Read the model definition and answer for the solid it produces. Units are mm, in the model's axes. A direction names the side the tool comes from. Coordinates: 2 decimals unless noted, no trailing zeros. Write each loop counter-clockwise with the first axis right and the second up, starting at its lowest first coordinate (ties: lowest second). Pieces come first, ordered by that corner, then holes. Notation, with made-up numbers: (-30.75, -3) -> (13.25, -3) arc R21 ccw to (13.25, 21) -> close; hole circle Ø11 at (-12.75, 55). An arc over 180 degrees is marked (long way). Answer as a JSON object with one key per item and string values. Group by question number.
(1) Which of the six approach directions +Z, -Z, +X, -X, +Y, -Y give full straight-line access (tool end or side, diameter ignored) to faces 1 (the face through (14.8, -8, 7.6)), 2 (the face through (22.5, -2, 42)), 3 (the face through (-19.791, 9.986, 10.607)), 4 (the face through (-5, 4, 14)), 5 (the face through (15, 16, 11))?
(2) Find section C-C (z = 10.5). Give the vertices of the cut face in (x, y).
(3) Straight lines are drawn through the part: L1, parallel to Z at x = 15, y = 0.25; L2, parallel to Z at x = 15, y = -5.5; L3, parallel to Z at x = -15, y = 10.2. For each, find the intervals that lie inside material, in ascending order.
(4) For a pull along X with two mould halves and no side action, classify faces 6 (the face through (8, -3, 15)), 7 (the face through (15, -11, 30)), 8 (the face through (-25, 12, 16)) as +X half, -X half, draft (parallel to the pull), parting line (faces both ways), or undercut.
(5) Find section D-D (x = 24.5). Give the vertices of the cut face in (y, z), then the cut area to 3 significant figures.
(6) Flat-ended cylindrical pins translate along their axes: P1, Ø6, axis at x = -19, z = 13.5, coming from the -Y side; P2, Ø4, axis at y = 14, z = 4.5, coming from the -X side; P3, Ø1.5, axis at y = -6, z = 17, coming from the -X side. Find the tip coordinate at first contact, or state that the pin passes through.
(7) Find section B-B (x = 15). Give the vertices of the cut face in (y, z).
from build123d import *

# Parameters (mm, degrees)
CYLINDER007_R         = 3.15
CYLINDER007_DEPTH     = 20
CYLINDER006_R         = 3.15
CYLINDER006_DEPTH     = 20
BOX010_W              = 20
BOX010_H              = 6.3
BOX010_DEPTH          = 1
BOX006_W              = 15
BOX006_H              = 27
BOX006_DEPTH          = 30
CHAMFER002001002_SIZE = 7
FILLET_R              = 12
CHAMFER002001003_SIZE = 4
CYLINDER009_R         = 6.5
CYLINDER009_DEPTH     = 19
CYLINDER008_R         = 3.25
CYLINDER008_DEPTH     = 19
CYLINDER004_R         = 3.15
CYLINDER004_DEPTH     = 36
CYLINDER005_R         = 7
CYLINDER005_DEPTH     = 36
BOX008_W              = 7.8
BOX008_H              = 1
BOX008_DEPTH          = 27
BOX009_W              = 24.5
BOX009_H              = 2
BOX009_DEPTH          = 7.3
CHAMFER002001008_SIZE = 1
BOX011_W              = 33
BOX011_H              = 3.5
BOX011_DEPTH          = 8
BOX012_W              = 20
BOX012_H              = 6
BOX012_DEPTH          = 27
CHAMFER002001007_SIZE = 3
BOX007_W              = 35
BOX007_H              = 23
BOX007_DEPTH          = 27
CHAMFER002001005_SIZE = 3
CHAMFER002001006_SIZE = 8
CHAMFER002001009_SIZE = 3.49
CHAMFER002001010_SIZE = 0.4


with BuildPart() as cylinder007:
    # Cylinder007 → Cylinder007 (new body)
    with BuildSketch(Plane(origin=(0, 0, 1), x_dir=(0, 0, 1), z_dir=(-1, 0, 0))):
        Circle(CYLINDER007_R)
    extrude(amount=CYLINDER007_DEPTH)


with BuildPart() as cylinder006:
    # Cylinder006 → Cylinder006 (new body)
    with BuildSketch(Plane.ZY):
        Circle(CYLINDER006_R)
    extrude(amount=CYLINDER006_DEPTH)


with BuildPart() as fusion003004:
    # Box010 → Box010 (new body)
    with BuildSketch(Plane(origin=(-20, -3.15, 0), x_dir=(1, 0, 0), z_dir=(0, 0, 1))):
        with Locations((10, 3.15)):
            Rectangle(BOX010_W, BOX010_H)
    extrude(amount=BOX010_DEPTH)

    # Fusion003004: union Cylinder007, Cylinder006
    add(cylinder007.part)
    add(cylinder006.part)


with BuildPart() as fusion003004_1:
    # Fusion003004 placement: moved
    add(fusion003004.part.moved(Location((25, 0, 45))))


with BuildPart() as cut004:
    # Box006 → Box006 (new body)
    with BuildSketch(Plane(origin=(7.5, -15, 27), x_dir=(1, 0, 0), z_dir=(0, 0, 1))):
        with Locations((7.5, 13.5)):
            Rectangle(BOX006_W, BOX006_H)
    extrude(amount=BOX006_DEPTH)

    # Chamfer002001002
    chamfer002001002_edges = [cut004.edges().sort_by_distance(p)[0] for p in [
        (15, -15, 27),
    ]]
    chamfer(chamfer002001002_edges, length=CHAMFER002001002_SIZE)

    # Fillet
    fillet_edges = [cut004.edges().sort_by_distance(p)[0] for p in [
        (15, 12, 57),
    ]]
    fillet(fillet_edges, radius=FILLET_R)

    # Chamfer002001003
    chamfer002001003_edges = [cut004.edges().sort_by_distance(p)[0] for p in [
        (15, -15, 57),
    ]]
    chamfer(chamfer002001003_edges, length=CHAMFER002001003_SIZE)

    # Cut004: cut Fusion003004
    add(fusion003004_1.part, mode=Mode.SUBTRACT)


with BuildPart() as cylinder009:
    # Cylinder009 → Cylinder009 (new body)
    with BuildSketch(Plane(origin=(-15, -8, 15), x_dir=(1, 0, 0), z_dir=(0, 1, 0))):
        Circle(CYLINDER009_R)
    extrude(amount=CYLINDER009_DEPTH)


with BuildPart() as cylinder008:
    # Cylinder008 → Cylinder008 (new body)
    with BuildSketch(Plane(origin=(-15, 0, 15), x_dir=(1, 0, 0), z_dir=(0, 1, 0))):
        Circle(CYLINDER008_R)
    extrude(amount=CYLINDER008_DEPTH)


with BuildPart() as cylinder004:
    # Cylinder004 → Cylinder004 (new body)
    with BuildSketch(Plane(origin=(15, -15, 15), x_dir=(1, 0, 0), z_dir=(0, 1, 0))):
        Circle(CYLINDER004_R)
    extrude(amount=CYLINDER004_DEPTH)


with BuildPart() as fusion003008:
    # Cylinder005 → Cylinder005 (new body)
    with BuildSketch(Plane(origin=(15, -34, 15), x_dir=(1, 0, 0), z_dir=(0, 1, 0))):
        Circle(CYLINDER005_R)
    extrude(amount=CYLINDER005_DEPTH)

    # Fusion003008: union Cylinder004
    add(cylinder004.part)


with BuildPart() as cube008:
    # Box008 → Box008 (new body)
    with BuildSketch(Plane(origin=(11.1, 15, 0), x_dir=(1, 0, 0), z_dir=(0, 0, 1))):
        with Locations((3.9, 0.5)):
            Rectangle(BOX008_W, BOX008_H)
    extrude(amount=BOX008_DEPTH)


with BuildPart() as fusion003010:
    # Box009 → Box009 (new body)
    with BuildSketch(Plane(origin=(-25, 14, 11.6), x_dir=(1, 0, 0), z_dir=(0, 0, 1))):
        with Locations((12.25, 1)):
            Rectangle(BOX009_W, BOX009_H)
    extrude(amount=BOX009_DEPTH)

    # Chamfer002001008
    chamfer002001008_edges = [fusion003010.edges().sort_by_distance(p)[0] for p in [
        (-12.75, 16, 11.6),
    ]]
    chamfer(chamfer002001008_edges, length=CHAMFER002001008_SIZE)

    # Fusion003010: union Cube008
    add(cube008.part)


with BuildPart() as cube011:
    # Box011 → Box011 (new body)
    with BuildSketch(Plane(origin=(-25, 11.5, 0), x_dir=(1, 0, 0), z_dir=(0, 0, 1))):
        with Locations((16.5, 1.75)):
            Rectangle(BOX011_W, BOX011_H)
    extrude(amount=BOX011_DEPTH)


with BuildPart() as chamfer002001007:
    # Box012 → Box012 (new body)
    with BuildSketch(Plane(origin=(-25, 9, 0), x_dir=(1, 0, 0), z_dir=(0, 0, 1))):
        with Locations((10, 3)):
            Rectangle(BOX012_W, BOX012_H)
    extrude(amount=BOX012_DEPTH)

    # Chamfer002001007
    chamfer002001007_edges = [chamfer002001007.edges().sort_by_distance(p)[0] for p in [
        (-25, 12, 27),
        (-25, 12, 0),
    ]]
    chamfer(chamfer002001007_edges, length=CHAMFER002001007_SIZE)


with BuildPart() as chamfer002001010:
    # Box007 → Box007 (new body)
    with BuildSketch(Plane(origin=(-5, -8, 0), x_dir=(1, 0, 0), z_dir=(0, 0, 1))):
        with Locations((17.5, 11.5)):
            Rectangle(BOX007_W, BOX007_H)
    extrude(amount=BOX007_DEPTH)

    # Chamfer002001005
    chamfer002001005_edges = [chamfer002001010.edges().sort_by_distance(p)[0] for p in [
        (30, -8, 13.5),
    ]]
    chamfer(chamfer002001005_edges, length=CHAMFER002001005_SIZE)

    # Chamfer002001006
    chamfer002001006_edges = [chamfer002001010.edges().sort_by_distance(p)[0] for p in [
        (-5, -8, 13.5),
    ]]
    chamfer(chamfer002001006_edges, length=CHAMFER002001006_SIZE)

    # Fusion003009: union Chamfer002001007
    add(chamfer002001007.part)

    # Cut005: cut Cube011
    add(cube011.part, mode=Mode.SUBTRACT)

    # Chamfer002001009
    chamfer002001009_edges = [chamfer002001010.edges().sort_by_distance(p)[0] for p in [
        (1.5, 15, 8),
    ]]
    chamfer(chamfer002001009_edges, length=CHAMFER002001009_SIZE)

    # Fusion003011: union Fusion003010
    add(fusion003010.part)

    # Cut006: cut Fusion003008
    add(fusion003008.part, mode=Mode.SUBTRACT)

    # Cut007: cut Cylinder008
    add(cylinder008.part, mode=Mode.SUBTRACT)

    # Cut008: cut Cylinder009
    add(cylinder009.part, mode=Mode.SUBTRACT)

    # Fusion003012: union Cut004
    add(cut004.part)

    # Chamfer002001010
    chamfer002001010_edges = [chamfer002001010.edges().sort_by_distance(p)[0] for p in [
        (8, 13.25, 0),
        (-7, 11.5, 0),
        (-13.5, 9, 0),
        (24.45, 15, 0),
        (30, 5, 0),
        (28.5, -6.5, 0),
        (15, -8, 0),
        (-1, -4, 0),
        (-5, 4.5, 0),
        (18.9, 15.5, 0),
        (11.1, 15.5, 0),
        (15, 16, 0),
        (9.55, 15, 0),
    ]]
    chamfer(chamfer002001010_edges, length=CHAMFER002001010_SIZE)


solid = chamfer002001010.part
Results below:
{
 "1": {"face 1": "-Z, +X, -X, -Y", "face 2": "+Z, +X, +Y, -Y", "face 3": "-Y", "face 4": "+Z, -Z, -X, -Y", "face 5": "+Z, -Z, +X, -X, +Y"},
 "2": {"outline": "(-25, 9) -> (-19.69, 9) -> (-19.69, 11) -> (-10.31, 11) -> (-10.31, 9) -> (-5, 9) -> (-5, 0) -> (3, -8) -> (9.64, -8) -> (9.64, 2) -> (20.36, 2) -> (20.36, -8) -> (27, -8) -> (30, -5) -> (30, 15) -> (18.9, 15) -> (18.9, 16) -> (11.1, 16) -> (11.1, 15) -> (8, 15) -> (8, 14.01) -> (-25, 14.01) -> close"},
 "3": {"L1": "z = 0 to 8, 22 to 41.86, 49.14 to 57", "L2": "z = 0 to 8, 22 to 57", "L3": "z = 0 to 8.5, 21.5 to 27"},
 "4": {"face 6": "undercut", "face 7": "draft", "face 8": "-X half"},
 "5": {"outline": "(-8, 0.4) -> (-7.6, 0) -> (14.6, 0) -> (15, 0.4) -> (15, 27) -> (-8, 27) -> close", "area": "621 mm2"},
 "6": {"P1": "stops at y = 9", "P2": "stops at x = 8", "P3": "stops at x = 0.25"},
 "7": {"outline": "(-15, 34) -> (-8, 27) -> (-8, 22) -> (2, 22) -> (2, 18.15) -> (16, 18.15) -> (16, 27) -> (12, 27) -> (12, 45) arc R12 ccw to (0, 57) -> (-11, 57) -> (-15, 53) -> close; (-8, 0.4) -> (-7.6, 0) -> (15.6, 0) -> (16, 0.4) -> (16, 11.85) -> (2, 11.85) -> (2, 8) -> (-8, 8) -> close; hole (-3.15, 45) arc R3.15 ccw to (3.15, 45) -> (3.15, 46) arc R3.15 ccw to (-3.15, 46) -> close"}
}
